```python
from build123d import *

# Parameters (mm, degrees)
F0_R      = 1.7
F0_R_2    = 4.1
F1_DEPTH  = 4.6
F2_R      = 6.8
F3_DEPTH  = 14
F3_FACE_R = 4.1
F4_DEPTH  = 10
F5_R      = 1


with BuildPart() as f1:
    # F0 (on Top) → F1 (new body)
    with BuildSketch(Plane.XY):
        with BuildLine():
            ThreePointArc((-15.6, -6.2), (-11.215938, -4.384062), (-9.4, 0))
            ThreePointArc((-9.4, 0), (-11.215938, 4.384062), (-15.6, 6.2))
            ThreePointArc((-15.6, 6.2), (-21.8, 0), (-15.6, -6.2))
        make_face()
        with Locations((-15.6, 0)):
            Circle(F0_R, mode=Mode.SUBTRACT)
        with BuildLine():
            ThreePointArc((-15.6, 6.2), (-11.215938, 4.384062), (-9.4, 0))
            ThreePointArc((-9.4, 0), (-11.215938, -4.384062), (-15.6, -6.2))
            Line((-15.6, -6.2), (-1.944236, -7.863202))
            ThreePointArc((-1.944236, -7.863202), (-8.1, 0), (-1.944236, 7.863202))
            Line((-1.944236, 7.863202), (-15.6, 6.2))
        make_face()
        with BuildLine():
            Line((0, 8.1), (-1.944236, 7.863202))
            ThreePointArc((-1.944236, 7.863202), (-8.1, 0), (-1.944236, -7.863202))
            Line((-1.944236, -7.863202), (0, -8.1))
            ThreePointArc((0, -8.1), (5.727565, -5.727565), (8.1, 0))
            ThreePointArc((8.1, 0), (5.727565, 5.727565), (0, 8.1))
        make_face()
        Circle(F0_R_2, mode=Mode.SUBTRACT)
        with BuildLine():
            ThreePointArc((0, 8.1), (-0.979302, 8.040583), (-1.944236, 7.863202))
            Line((-1.944236, 7.863202), (0, 8.1))
        make_face()
        with BuildLine():
            Line((0, -8.1), (-1.944236, -7.863202))
            ThreePointArc((-1.944236, -7.863202), (-0.979302, -8.040583), (0, -8.1))
        make_face()
    extrude(amount=F1_DEPTH)

    # F2 (on face) → F3 (join)
    with BuildSketch(Plane.XY.offset(4.6)):
        Circle(F2_R)
    extrude(amount=F3_DEPTH)

    # F3_face (on face) → F4 (cut)
    with BuildSketch(Plane(origin=(0, 0, 4.6), x_dir=(1, 0, 0), z_dir=(0, 0, -1))):
        Circle(F3_FACE_R)
    extrude(amount=-F4_DEPTH, mode=Mode.SUBTRACT)

    # F5
    f5_edges = [f1.edges().sort_by_distance(p)[0] for p in [
        (-6.8, 0, 4.6),
        (-6.8, 0, 18.6),
    ]]
    fillet(f5_edges, radius=F5_R)


solid = f1.part
```
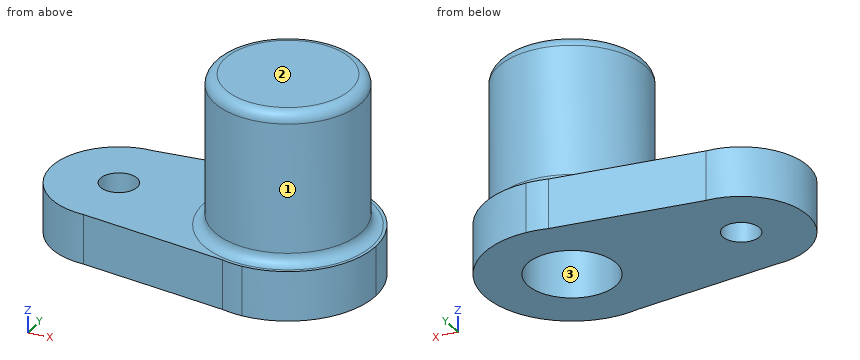
Input: part model. Units: mm. Frame: model coordinates. Face numbers are marked on the shaded views. Coordinates: 2 decimals unless noted, no trailing zeros. Loops run counter-clockwise (first coordinate to the right, second up) from the corner with the lowest first, then second, coordinate; pieces in that order, holes last. Notation, with made-up numbers: M 12,22.5 L 69,22.5 A17 ccw 69,46.5 Z; hole C -12.75,-5.75 d7. An arc over 180 degrees is marked long. Use a Markdown table: item, result. Add a question column.
1) Line query: L1, parallel to Y at x = -15.6, z = 2.55; L2, parallel to Y at x = 0, z = 7.5; L3, parallel to Z at x = -16.25, y = -3. Output: solid intervals per line, ascending. Write a range as from..to.
2) Section B-B, the plane x = -16.5. Return the cut outline in (y, z).
3) Section C-C, the plane z = 10.5. Return the cut outline in (x, y), plus the area to 3 significant figures.
4) Pin query (flat end, axial travel): P1, Ø8, axis at x = -1, z = 8.5, coming from the -Y side; P2, Ø1, axis at y = -4, z = 2, coming from the -X side; P3, Ø2.5, axis at x = -1.5, y = -0.5, coming from the -Z side; P4, Ø6, axis at y = -5, z = 4, coming from the +X side. Return the tip coordinate at first contact, or that it passes through.
5) Section A-A, the plane z = 2. Return the cut outline in (x, y), plus the area to 3 significant figures.
6) Draft query along Y for the marked faces 1, 2 and 3. Return one class per face: +Y half, -Y half, draft (parallel to the pull), parting line (faces both ways), or undercut.
7) Section D-D, the plane x = -19.5. Return the cut outline in (y, z), plus the area to 3 significant figures.
Answer below:
| question | item | result |
|---|---|---|
| 1 | L1 | -6.2..-1.7, 1.7..6.2 |
| 1 | L2 | -6.8..-4.1, 4.1..6.8 |
| 1 | L3 | 0..4.6 |
| 2 | outline | M -6.13,0 L -1.44,0 L -1.44,4.6 L -6.13,4.6 Z; M 1.44,0 L 6.13,0 L 6.13,4.6 L 1.44,4.6 Z |
| 3 | outline | C 0,0 d13.6; hole C 0,0 d8.2 |
| 3 | area | 92.5 mm2 |
| 4 | P1 | y = -8.1 |
| 4 | P2 | x = -20.72 |
| 4 | P3 | z = 14.6 |
| 4 | P4 | x = 7.85 |
| 5 | outline | M -15.6,-6.2 L -1.94,-7.86 A8.1 ccw 0,-8.1 A8.1 ccw 0,8.1 A8.1 ccw -1.94,7.86 L -15.6,6.2 A6.2 ccw Z; hole C -15.6,0 d3.4; hole C 0,0 d8.2 |
| 5 | area | 325 mm2 |
| 6 | face 1 | parting line |
| 6 | face 2 | draft |
| 6 | face 3 | undercut |
| 7 | outline | M -4.82,0 L 4.82,0 L 4.82,4.6 L -4.82,4.6 Z |
| 7 | area | 44.3 mm2 |
